Source: CAD feature listing. Evaluate the final solid. Frame: model axes, mm. Face numbers are marked on the shaded views. A direction names the side the tool comes from. Coordinates: 2 decimals unless noted, no trailing zeros. Write each loop counter-clockwise with the first axis right and the second up, starting at its lowest first coordinate (ties: lowest second). Pieces come first, ordered by that corner, then holes. Notation, with made-up numbers: (74.25, -20.75) -> (132.25, -20.75) arc R26 cw to (132.25, 6.25) -> close; hole circle Ø1 at (62, 16). An arc over 180 degrees is marked (long way). Write item = value, one per line.
from build123d import *

# Parameters (mm, degrees)
EXTRUDE_1_DEPTH = 20
CHAMFER_1_SIZE  = 20


with BuildPart() as part:
    # 草图1 → 凸台-拉伸1 (new body)
    with BuildSketch(Plane.XY):
        with BuildLine():
            Line((0, 0), (19, 0))
            Line((19, 0), (19, -80))
            ThreePointArc((19, -80), (27.786796564, -101.213203436), (49, -110))
            Line((49, -110), (100, -110))
            Line((100, -110), (100, -190))
            Line((100, -190), (0, -190))
            Line((0, -190), (0, 0))
        make_face()
    extrude(amount=EXTRUDE_1_DEPTH)

    # 倒角1
    chamfer_1_edges = [part.edges().sort_by_distance(p)[0] for p in [
        (100, -190, 10),
        (0, -190, 10),
    ]]
    chamfer(chamfer_1_edges, length=CHAMFER_1_SIZE)


solid = part.part
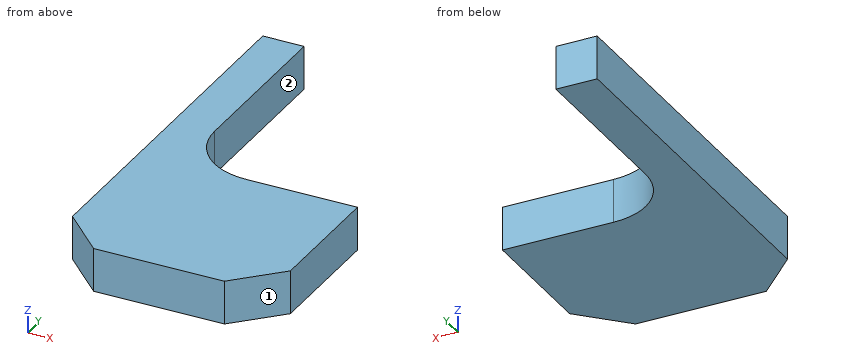
1) Cut plane B-B, the plane y = -178. Output: boundary loops of the cut face in (x, z), and give its area (3 significant figures).
Answer block:
outline = (8, 0) -> (92, 0) -> (92, 20) -> (8, 20) -> close
area = 1,680 mm2
2) Material intervals for probe 1 along X at (y, z) = (-48, 12.75); probe 2 along Y at (x, z) = (52.5, 11.5); probe 3 along X at (y, z) = (-87.5, 6.25), sorted ascending. Write a range as [from, to].
Answer block:
probe_1 = [0, 19]
probe_2 = [-190, -110]
probe_3 = [0, 19.95]
3) Cut plane C-C, the plane x = 12. Output: boundary loops of the cut face in (y, z), and give its area (3 significant figures).
Answer block:
outline = (-182, 0) -> (0, 0) -> (0, 20) -> (-182, 20) -> close
area = 3,640 mm2
4) Reachability of the marked faces 1 and 2 from +Z, -Z, +X, -X, +Y, -Y: full face, straight path, thin tool, end or side. Return the list, or none.
Answer block:
face_1 = +Z, -Z, +X, -Y
face_2 = +Z, -Z, +X, +Y
5) First-contact query: pin 1 Ø1 at (y, z) = (-60, 7.5) entering from +X. Flat tip, straight axial feed; report the tip coordinate or a pass-through.
Answer block:
pin_1 = 19
6) Cut plane A-A, the plane z = 15.5. Output: boundary loops of the cut face in (x, y), and give its area (3 significant figures).
Answer block:
outline = (0, -170) -> (20, -190) -> (80, -190) -> (100, -170) -> (100, -110) -> (49, -110) arc R30 cw to (19, -80) -> (19, 0) -> (0, 0) -> close
area = 9,880 mm2
